Here's how the part is built. I have some questions about the finished solid (model axes, mm). Face numbers are marked on the shaded views. A direction names the side the tool comes from. Round coordinates to 2 decimals unless told otherwise and drop trailing zeros. Write each loop counter-clockwise with the first axis right and the second up, starting at its lowest first coordinate (ties: lowest second). Pieces come first, ordered by that corner, then holes. Notation, with made-up numbers: (74, -39.5) -> (127, -39.5) arc R25 cw to (127, -12.5) -> close; hole circle Ø2 at (-0.75, 87.25). An arc over 180 degrees is marked (long way). Answer in a Markdown table with one row per item.
from build123d import *

# Parameters (mm, degrees)
SKETCH3_W           = 58
SKETCH3_H           = 16
BOSS_EXTRUDE2_DEPTH = 30
CUT_EXTRUDE2_REACH  = 3
SKETCH4_R           = 2.5
CUT_EXTRUDE6_REACH  = 3
SKETCH7_W           = 22
SKETCH7_H           = 12
BOSS_EXTRUDE4_REACH = 16
SKETCH9_W           = 5
SKETCH9_H           = 1
CHAMFER1_SIZE       = 5
SKETCH10_R          = 1.6
SKETCH10_W          = 9
SKETCH10_H          = 9
BOSS_EXTRUDE5_DEPTH = 3
CUT_EXTRUDE8_DEPTH  = 1.5
CUT_EXTRUDE9_REACH  = 69
SKETCH12_W          = 3.5
SKETCH12_H          = 1
CUT_EXTRUDE10_REACH = 18
SKETCH13_W          = 9
SKETCH13_H          = 1.1
CUT_EXTRUDE12_REACH = 18
SKETCH14_W          = 8
SKETCH14_H          = 5


with BuildPart() as part:
    # Sketch3 → Boss-Extrude2 (new body)
    with BuildSketch(Plane(origin=(0, 0, 0), x_dir=(0, 0, -1), z_dir=(1, 0, 0))):
        with Locations((29, 8)):
            Rectangle(SKETCH3_W, SKETCH3_H)
        Polygon((1, 1), (19, 1), (19, 2), (20, 2), (20, 1), (38, 1), (38, 2), (39, 2), (39, 1), (57, 1), (57, 15), (1, 15), align=None, mode=Mode.SUBTRACT)
    extrude(amount=BOSS_EXTRUDE2_DEPTH)

    # Sketch4 → Cut-Extrude2 (cut, up to next)
    with BuildSketch(Plane(origin=(0, 1, 0), x_dir=(1, 0, 0), z_dir=(0, 1, 0)), mode=Mode.PRIVATE) as cut_extrude2_sk1:
        with Locations(Location((22, 54.5, 0), (0, 0, 270))):  # turned: the seam where the file's is
            Circle(SKETCH4_R)
    cut_extrude2_tool1 = extrude(cut_extrude2_sk1.sketch, amount=-CUT_EXTRUDE2_REACH, mode=Mode.PRIVATE) & part.part
    add(cut_extrude2_tool1.solids().sort_by_distance((22, 1, -54.5))[0], mode=Mode.SUBTRACT)
    # Sketch4 → Cut-Extrude2 (cut, up to next)
    with BuildSketch(Plane(origin=(0, 1, 0), x_dir=(1, 0, 0), z_dir=(0, 1, 0)), mode=Mode.PRIVATE) as cut_extrude2_sk2:
        with Locations(Location((8, 54.5, 0), (0, 0, 270))):  # turned: the seam where the file's is
            Circle(SKETCH4_R)
    cut_extrude2_tool2 = extrude(cut_extrude2_sk2.sketch, amount=-CUT_EXTRUDE2_REACH, mode=Mode.PRIVATE) & part.part
    add(cut_extrude2_tool2.solids().sort_by_distance((8, 1, -54.5))[0], mode=Mode.SUBTRACT)
    # Sketch4 → Cut-Extrude2 (cut, up to next)
    with BuildSketch(Plane(origin=(0, 1, 0), x_dir=(1, 0, 0), z_dir=(0, 1, 0)), mode=Mode.PRIVATE) as cut_extrude2_sk3:
        with Locations(Location((8, 35.5, 0), (0, 0, 270))):  # turned: the seam where the file's is
            Circle(SKETCH4_R)
    cut_extrude2_tool3 = extrude(cut_extrude2_sk3.sketch, amount=-CUT_EXTRUDE2_REACH, mode=Mode.PRIVATE) & part.part
    add(cut_extrude2_tool3.solids().sort_by_distance((8, 1, -35.5))[0], mode=Mode.SUBTRACT)
    # Sketch4 → Cut-Extrude2 (cut, up to next)
    with BuildSketch(Plane(origin=(0, 1, 0), x_dir=(1, 0, 0), z_dir=(0, 1, 0)), mode=Mode.PRIVATE) as cut_extrude2_sk4:
        with Locations(Location((22, 35.5, 0), (0, 0, 270))):  # turned: the seam where the file's is
            Circle(SKETCH4_R)
    cut_extrude2_tool4 = extrude(cut_extrude2_sk4.sketch, amount=-CUT_EXTRUDE2_REACH, mode=Mode.PRIVATE) & part.part
    add(cut_extrude2_tool4.solids().sort_by_distance((22, 1, -35.5))[0], mode=Mode.SUBTRACT)
    # Sketch4 → Cut-Extrude2 (cut, up to next)
    with BuildSketch(Plane(origin=(0, 1, 0), x_dir=(1, 0, 0), z_dir=(0, 1, 0)), mode=Mode.PRIVATE) as cut_extrude2_sk5:
        with Locations(Location((8, 16.5, 0), (0, 0, 270))):  # turned: the seam where the file's is
            Circle(SKETCH4_R)
    cut_extrude2_tool5 = extrude(cut_extrude2_sk5.sketch, amount=-CUT_EXTRUDE2_REACH, mode=Mode.PRIVATE) & part.part
    add(cut_extrude2_tool5.solids().sort_by_distance((8, 1, -16.5))[0], mode=Mode.SUBTRACT)
    # Sketch4 → Cut-Extrude2 (cut, up to next)
    with BuildSketch(Plane(origin=(0, 1, 0), x_dir=(1, 0, 0), z_dir=(0, 1, 0)), mode=Mode.PRIVATE) as cut_extrude2_sk6:
        with Locations(Location((22, 16.5, 0), (0, 0, 270))):  # turned: the seam where the file's is
            Circle(SKETCH4_R)
    cut_extrude2_tool6 = extrude(cut_extrude2_sk6.sketch, amount=-CUT_EXTRUDE2_REACH, mode=Mode.PRIVATE) & part.part
    add(cut_extrude2_tool6.solids().sort_by_distance((22, 1, -16.5))[0], mode=Mode.SUBTRACT)

    # Sketch7 → Cut-Extrude6 (cut, up to next)
    with BuildSketch(Plane.XY.offset(-57), mode=Mode.PRIVATE) as cut_extrude6_sk1:
        with Locations((16, 9)):
            Rectangle(SKETCH7_W, SKETCH7_H)
    cut_extrude6_tool1 = extrude(cut_extrude6_sk1.sketch, amount=-CUT_EXTRUDE6_REACH, mode=Mode.PRIVATE) & part.part
    add(cut_extrude6_tool1.solids().sort_by_distance((16, 9, -57))[0], mode=Mode.SUBTRACT)

    # Sketch9 → Boss-Extrude4 (add, up to next)
    with BuildSketch(Plane(origin=(0, 2, 0), x_dir=(1, 0, 0), z_dir=(0, 1, 0)), mode=Mode.PRIVATE) as boss_extrude4_sk1:
        with Locations((15, 19.5)):
            Rectangle(SKETCH9_W, SKETCH9_H)
    boss_extrude4_tool1 = extrude(boss_extrude4_sk1.sketch, amount=BOSS_EXTRUDE4_REACH, mode=Mode.PRIVATE) - part.part
    add(boss_extrude4_tool1.solids().sort_by_distance((15, 2, -19.5))[0])
    # Sketch9 → Boss-Extrude4 (add, up to next)
    with BuildSketch(Plane(origin=(0, 2, 0), x_dir=(1, 0, 0), z_dir=(0, 1, 0)), mode=Mode.PRIVATE) as boss_extrude4_sk2:
        with Locations((15, 38.5)):
            Rectangle(SKETCH9_W, SKETCH9_H)
    boss_extrude4_tool2 = extrude(boss_extrude4_sk2.sketch, amount=BOSS_EXTRUDE4_REACH, mode=Mode.PRIVATE) - part.part
    add(boss_extrude4_tool2.solids().sort_by_distance((15, 2, -38.5))[0])

    # Chamfer1
    chamfer1_edges = [part.edges().sort_by_distance(p)[0] for p in [
        (12.5, 2, -19.5),
        (12.5, 2, -38.5),
    ]]
    chamfer(chamfer1_edges, length=CHAMFER1_SIZE)

    # Sketch10 → Boss-Extrude5 (add)
    with BuildSketch(Plane.XZ):
        Polygon((19.5, 0), (5.303847577, 0), (10.5, 9), (19.5, 9), align=None)
        with Locations(Location((15, 4.5, 0), (0, 0, 270))):  # turned: the seam where the file's is
            Circle(SKETCH10_R, mode=Mode.SUBTRACT)
        with Locations((15, -62.5)):
            Rectangle(SKETCH10_W, SKETCH10_H)
        with Locations(Location((15, -62.5, 0), (0, 0, 270))):  # turned: the seam where the file's is
            Circle(SKETCH10_R, mode=Mode.SUBTRACT)
    extrude(amount=-BOSS_EXTRUDE5_DEPTH)

    # Sketch11 → Cut-Extrude8 (cut)
    with BuildSketch(Plane(origin=(0, 3, 0), x_dir=(1, 0, 0), z_dir=(0, 1, 0))):
        Polygon((11.766838493, 62.5), (13.383419246, 59.7), (16.616580754, 59.7), (18.233161507, 62.5), (16.616580754, 65.3), (13.383419246, 65.3), align=None)
        Polygon((11.766838493, -4.5), (13.383419246, -7.3), (16.616580754, -7.3), (18.233161507, -4.5), (16.616580754, -1.7), (13.383419246, -1.7), align=None)
    extrude(amount=-CUT_EXTRUDE8_DEPTH, mode=Mode.SUBTRACT)

    # Sketch12 → Cut-Extrude9 (cut, up to next)
    with BuildSketch(Plane.XY, mode=Mode.PRIVATE) as cut_extrude9_sk1:
        with Locations((1.75, 8)):
            Rectangle(SKETCH12_W, SKETCH12_H)
    cut_extrude9_tool1 = extrude(cut_extrude9_sk1.sketch, amount=-CUT_EXTRUDE9_REACH, mode=Mode.PRIVATE) & part.part
    add(cut_extrude9_tool1.solids().sort_by_distance((1.75, 8, 0))[0], mode=Mode.SUBTRACT)
    # Sketch12 → Cut-Extrude9 (cut, up to next)
    with BuildSketch(Plane.XY, mode=Mode.PRIVATE) as cut_extrude9_sk2:
        with Locations((28.25, 8)):
            Rectangle(SKETCH12_W, SKETCH12_H)
    cut_extrude9_tool2 = extrude(cut_extrude9_sk2.sketch, amount=-CUT_EXTRUDE9_REACH, mode=Mode.PRIVATE) & part.part
    add(cut_extrude9_tool2.solids().sort_by_distance((28.25, 8, 0))[0], mode=Mode.SUBTRACT)

    # Sketch13 → Cut-Extrude10 (cut, up to next)
    with BuildSketch(Plane.XZ, mode=Mode.PRIVATE) as cut_extrude10_sk1:
        with Locations((15, -66.45)):
            Rectangle(SKETCH13_W, SKETCH13_H)
    cut_extrude10_tool1 = extrude(cut_extrude10_sk1.sketch, amount=-CUT_EXTRUDE10_REACH, mode=Mode.PRIVATE) & part.part
    add(cut_extrude10_tool1.solids().sort_by_distance((15, 0, -66.45))[0], mode=Mode.SUBTRACT)

    # Sketch14 → Cut-Extrude12 (cut, up to next)
    with BuildSketch(Plane(origin=(0, 16, 0), x_dir=(1, 0, 0), z_dir=(0, 1, 0)), mode=Mode.PRIVATE) as cut_extrude12_sk1:
        with BuildLine():
            Line((12.898979486, 57), (3.101020514, 57))
            ThreePointArc((3.101020514, 57), (8, 49), (12.898979486, 57))
        make_face()
    cut_extrude12_tool1 = extrude(cut_extrude12_sk1.sketch, amount=-CUT_EXTRUDE12_REACH, mode=Mode.PRIVATE) & part.part
    add(cut_extrude12_tool1.solids().sort_by_distance((8, 16, -53.441303))[0], mode=Mode.SUBTRACT)
    # Sketch14 → Cut-Extrude12 (cut, up to next)
    with BuildSketch(Plane(origin=(0, 16, 0), x_dir=(1, 0, 0), z_dir=(0, 1, 0)), mode=Mode.PRIVATE) as cut_extrude12_sk2:
        with BuildLine():
            Line((26.898979486, 57), (17.101020514, 57))
            ThreePointArc((17.101020514, 57), (22, 49), (26.898979486, 57))
        make_face()
    cut_extrude12_tool2 = extrude(cut_extrude12_sk2.sketch, amount=-CUT_EXTRUDE12_REACH, mode=Mode.PRIVATE) & part.part
    add(cut_extrude12_tool2.solids().sort_by_distance((22, 16, -53.441303))[0], mode=Mode.SUBTRACT)
    # Sketch14 → Cut-Extrude12 (cut, up to next)
    with BuildSketch(Plane(origin=(0, 16, 0), x_dir=(1, 0, 0), z_dir=(0, 1, 0)), mode=Mode.PRIVATE) as cut_extrude12_sk3:
        with BuildLine():
            Line((26.898979486, 38), (17.101020514, 38))
            ThreePointArc((17.101020514, 38), (22, 30), (26.898979486, 38))
        make_face()
    cut_extrude12_tool3 = extrude(cut_extrude12_sk3.sketch, amount=-CUT_EXTRUDE12_REACH, mode=Mode.PRIVATE) & part.part
    add(cut_extrude12_tool3.solids().sort_by_distance((22, 16, -34.441303))[0], mode=Mode.SUBTRACT)
    # Sketch14 → Cut-Extrude12 (cut, up to next)
    with BuildSketch(Plane(origin=(0, 16, 0), x_dir=(1, 0, 0), z_dir=(0, 1, 0)), mode=Mode.PRIVATE) as cut_extrude12_sk4:
        with BuildLine():
            Line((12.898979486, 38), (3.101020514, 38))
            ThreePointArc((3.101020514, 38), (8, 30), (12.898979486, 38))
        make_face()
    cut_extrude12_tool4 = extrude(cut_extrude12_sk4.sketch, amount=-CUT_EXTRUDE12_REACH, mode=Mode.PRIVATE) & part.part
    add(cut_extrude12_tool4.solids().sort_by_distance((8, 16, -34.441303))[0], mode=Mode.SUBTRACT)
    # Sketch14 → Cut-Extrude12 (cut, up to next)
    with BuildSketch(Plane(origin=(0, 16, 0), x_dir=(1, 0, 0), z_dir=(0, 1, 0)), mode=Mode.PRIVATE) as cut_extrude12_sk5:
        with BuildLine():
            Line((26.898979486, 19), (17.101020514, 19))
            ThreePointArc((17.101020514, 19), (22, 11), (26.898979486, 19))
        make_face()
    cut_extrude12_tool5 = extrude(cut_extrude12_sk5.sketch, amount=-CUT_EXTRUDE12_REACH, mode=Mode.PRIVATE) & part.part
    add(cut_extrude12_tool5.solids().sort_by_distance((22, 16, -15.441303))[0], mode=Mode.SUBTRACT)
    # Sketch14 → Cut-Extrude12 (cut, up to next)
    with BuildSketch(Plane(origin=(0, 16, 0), x_dir=(1, 0, 0), z_dir=(0, 1, 0)), mode=Mode.PRIVATE) as cut_extrude12_sk6:
        with BuildLine():
            Line((12.898979486, 19), (3.101020514, 19))
            ThreePointArc((3.101020514, 19), (8, 11), (12.898979486, 19))
        make_face()
    cut_extrude12_tool6 = extrude(cut_extrude12_sk6.sketch, amount=-CUT_EXTRUDE12_REACH, mode=Mode.PRIVATE) & part.part
    add(cut_extrude12_tool6.solids().sort_by_distance((8, 16, -15.441303))[0], mode=Mode.SUBTRACT)
    # Sketch14 → Cut-Extrude12 (cut, up to next)
    with BuildSketch(Plane(origin=(0, 16, 0), x_dir=(1, 0, 0), z_dir=(0, 1, 0)), mode=Mode.PRIVATE) as cut_extrude12_sk7:
        with Locations((15, 41.5)):
            Rectangle(SKETCH14_W, SKETCH14_H)
    cut_extrude12_tool7 = extrude(cut_extrude12_sk7.sketch, amount=-CUT_EXTRUDE12_REACH, mode=Mode.PRIVATE) & part.part
    add(cut_extrude12_tool7.solids().sort_by_distance((15, 16, -41.5))[0], mode=Mode.SUBTRACT)
    # Sketch14 → Cut-Extrude12 (cut, up to next)
    with BuildSketch(Plane(origin=(0, 16, 0), x_dir=(1, 0, 0), z_dir=(0, 1, 0)), mode=Mode.PRIVATE) as cut_extrude12_sk8:
        with Locations((15, 22.5)):
            Rectangle(SKETCH14_W, SKETCH14_H)
    cut_extrude12_tool8 = extrude(cut_extrude12_sk8.sketch, amount=-CUT_EXTRUDE12_REACH, mode=Mode.PRIVATE) & part.part
    add(cut_extrude12_tool8.solids().sort_by_distance((15, 16, -22.5))[0], mode=Mode.SUBTRACT)
    # Sketch14 → Cut-Extrude12 (cut, up to next)
    with BuildSketch(Plane(origin=(0, 16, 0), x_dir=(1, 0, 0), z_dir=(0, 1, 0)), mode=Mode.PRIVATE) as cut_extrude12_sk9:
        with Locations((15, 3.5)):
            Rectangle(SKETCH14_W, SKETCH14_H)
    cut_extrude12_tool9 = extrude(cut_extrude12_sk9.sketch, amount=-CUT_EXTRUDE12_REACH, mode=Mode.PRIVATE) & part.part
    add(cut_extrude12_tool9.solids().sort_by_distance((15, 16, -3.5))[0], mode=Mode.SUBTRACT)


solid = part.part
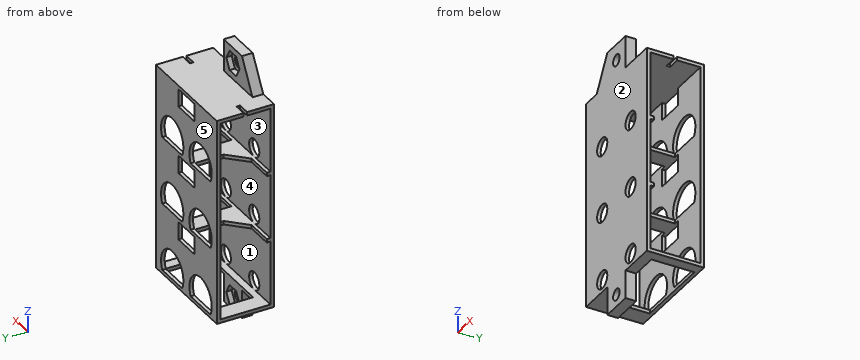
1) I want a section at D-D, the plane x = 15. Count the separate pieces of the cut face and the enclosed holes in it, and give its area (3 significant figures).
Response:
| item | result |
|---|---|
| separate pieces | 4 |
| enclosed holes | 0 |
| area | 169 mm^2 |
2) I want a section at B-B, the plane y = 4.5. List the corners of the cut face in (x, z) for me.
Response:
| item | result |
|---|---|
| outline | (0, -58) -> (5, -58) -> (5, -57) -> (0, -57) -> close; (0, -1) -> (30, -1) -> (30, 0) -> (0, 0) -> close; (10, -39) -> (17.5, -39) -> (17.5, -38) -> (10, -38) -> close; (10, -20) -> (17.5, -20) -> (17.5, -19) -> (10, -19) -> close; (27, -58) -> (30, -58) -> (30, -57) -> (27, -57) -> close |
3) For pin 1 (7.5 mm diameter, centred on x = 18, y = 11.5, fed in from +Z); pin 2 (1.1 mm diameter, centred on y = 9, z = -38.5, fed in from -X); pin 3 (7.5 mm diameter, centred on x = 21, y = 8, fed in from -Z), each with a flat end and sliding along its axis, tell me the tip position at first contact or that it passes through.
Response:
| item | result |
|---|---|
| pin 1 | stops at z = 0 |
| pin 2 | stops at x = 12.5 |
| pin 3 | stops at z = -39 |
4) We'd pull the mould along Z, two halves only. Please class the marked faces 1, 2 and 3: +Z half, -Z half, draft (parallel to the pull), parting line (faces both ways), or undercut.
Response:
| item | result |
|---|---|
| face 1 | undercut |
| face 2 | draft |
| face 3 | undercut |
5) I need wall thicknesses on line 1 (Z direction, x = 3.5, y = 1.5); line 2 (X direction, y = 15.3, z = -54.5); line 3 (Z direction, x = 22, y = 15.55). Which ranges of each line are inside material? Lowest first, please. Write a range as [from, to].
Response:
| item | result |
|---|---|
| line 1 | z = [-58, -57], [-39, -38], [-20, -19], [-1, 0] |
| line 2 | x = [0, 2.5], [13.5, 16.5], [27.5, 30] |
| line 3 | z = [-58, -57], [-49, -38], [-30, -19], [-11, 0] |
6) I want a section at C-C, the plane z = -28. List the corners of the cut face in (x, y) for me, and give its area (3 significant figures).
Response:
| item | result |
|---|---|
| outline | (0, 0) -> (30, 0) -> (30, 1) -> (0, 1) -> close; (0, 15) -> (30, 15) -> (30, 16) -> (0, 16) -> close |
| area | 60.0 mm^2 |
7) Which directions (+Z, -Z, +X, -X, +Y, -Y) give clear straight access to the entire face, cutting with the end or side of a thin tool? Please do the marked faces 4 and 5.
Response:
| item | result |
|---|---|
| face 4 | +X, -X |
| face 5 | +Z, -Z, +X, -X, +Y |
8) I want a section at A-A, the plane z = -40. List the corners of the cut face in (x, y) for me.
Response:
| item | result |
|---|---|
| outline | (0, 0) -> (30, 0) -> (30, 1) -> (0, 1) -> close; (0, 15) -> (11, 15) -> (11, 16) -> (0, 16) -> close; (19, 15) -> (30, 15) -> (30, 16) -> (19, 16) -> close |
